```python
from build123d import *

# Parameters (mm, degrees)
SKETCH_1_W           = 2000
SKETCH_1_H           = 262
EXTRUDE_1_DEPTH      = 200
SKETCH_5_W           = 232
SKETCH_5_H           = 238
SKETCH_5_W_2         = 488
CUT_EXTRUDE_10_DEPTH = 2027.979032945
SKETCH_7_W           = 2000
SKETCH_7_H           = 12
EXTRUDE_13_DEPTH     = 260


with BuildPart() as part:
    # 草图1 → 拉伸1 (new body)
    with BuildSketch(Plane.XY):
        with Locations((1000, 131)):
            Rectangle(SKETCH_1_W, SKETCH_1_H)
    extrude(amount=EXTRUDE_1_DEPTH)

    # 草图5 → 拉伸10 (cut, through all)
    with BuildSketch(Plane.XY.offset(200)):
        with Locations((128, 131)):
            Rectangle(SKETCH_5_W, SKETCH_5_H)
        with Locations((500, 131)):
            Rectangle(SKETCH_5_W_2, SKETCH_5_H)
        with Locations((1000, 131)):
            Rectangle(SKETCH_5_W_2, SKETCH_5_H)
        with Locations((1500, 131)):
            Rectangle(SKETCH_5_W_2, SKETCH_5_H)
        with Locations((1872, 131)):
            Rectangle(SKETCH_5_W, SKETCH_5_H)
    extrude(amount=-CUT_EXTRUDE_10_DEPTH, mode=Mode.SUBTRACT)

    # 草图7 → 拉伸13 (add)
    with BuildSketch(Plane.XZ):
        with Locations((1000, 100)):
            Rectangle(SKETCH_7_W, SKETCH_7_H)
    extrude(amount=-EXTRUDE_13_DEPTH)


solid = part.part
```
Here's how the part is built. I have some questions about the finished solid (model axes, mm). A direction names the side the tool comes from. Coordinates: 2 decimals unless noted, no trailing zeros. Order: outer loops, then holes, each group sorted by start corner. A loop starts at its lowest first (then second) coordinate and runs counter-clockwise, first axis right, second up. Notation, with made-up numbers: (86.25, 38) - (124.25, 38) arc R14 ccw to (124.25, 42) - close; hole circle Ø5 at (49, 55). An arc over 180 degrees is marked (long way). One line per question, with ' | ' between items.
(1) If we mould it in two halves opening along X, with no side actions, what happens to faces 4 (the flat face through (773, 5, 0)), 5 (the flat face through (1744, 129, 154))? For each: pulls with the +X half, pulls with the -X half, needs draft (parallel to the pull), parting line crosses it, or undercut.
Report:
face 4: needs draft | face 5: undercut
(2) If I drill on L1, parallel to X at y = 204, z = 145; L2, parallel to Y at x = 526, z = 92.5; L3, parallel to Z at x = 1708.5, y = 167, over which ranges is the centre line in solid material (lowest first)?
Report:
L1: x = 0 to 12, 244 to 256, 744 to 756, 1244 to 1256, 1744 to 1756, 1988 to 2000 | L2: y = 0 to 12, 250 to 262 | L3: z = 94 to 106
(3) Suppose I cut it at B-B on x = 327.5. List the corners of the cut face in (y, z) for me.
Report:
outline: (0, 0) - (12, 0) - (12, 94) - (250, 94) - (250, 0) - (262, 0) - (262, 200) - (250, 200) - (250, 106) - (12, 106) - (12, 200) - (0, 200) - close
(4) Will this pin go through, and if not, where does the flat tip stop? pin 1 (10 mm diameter, centred on x = 1115, y = 72, fed in from +Z).
Report:
pin 1: stops at z = 106
(5) For faces 1 (the flat face through (256, 129, 154)), 2 (the flat face through (986, 0, 101)), 3 (the flat face through (126, 12, 48)), which set-ups out of +Z, -Z, +X, -X, +Y, -Y let a thin tool reach every point of the face, with its end or its side?
Report:
face 1: +Z | face 2: +Z, -Z, +X, -X, -Y | face 3: -Z
(6) Suppose I cut it at A-A on z = 74.5. List the corners of the cut face in (x, y) for me, and give its area (3 significant figures).
Report:
outline: (0, 0) - (2000, 0) - (2000, 262) - (0, 262) - close; hole (12, 12) - (244, 12) - (244, 250) - (12, 250) - close; hole (256, 12) - (744, 12) - (744, 250) - (256, 250) - close; hole (756, 12) - (1244, 12) - (1244, 250) - (756, 250) - close; hole (1256, 12) - (1744, 12) - (1744, 250) - (1256, 250) - close; hole (1756, 12) - (1988, 12) - (1988, 250) - (1756, 250) - close | area: 65,100 mm2
